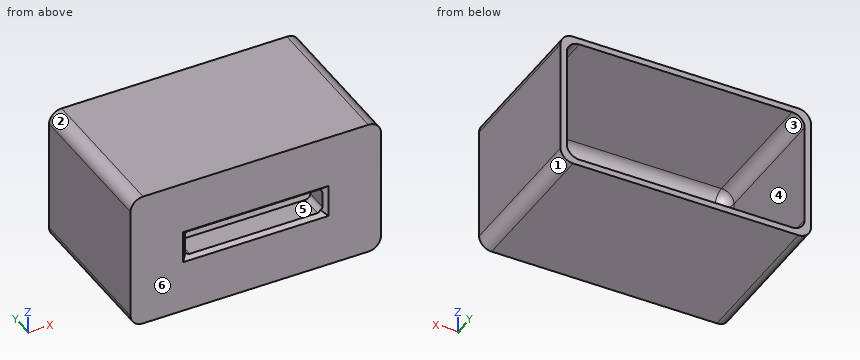
```python
from build123d import *

# Parameters (mm, degrees)
SKETCH1_W           = 200
SKETCH1_H           = 110
BOSS_EXTRUDE1_DEPTH = 6
SKETCH2_W           = 200
SKETCH2_H           = 110
SKETCH2_W_2         = 190
SKETCH2_H_2         = 100
BOSS_EXTRUDE2_DEPTH = 114
SKETCH3_W           = 110
SKETCH3_H           = 20
CUT_EXTRUDE1_DEPTH  = 256.139177705
SKETCH4_W           = 120
SKETCH4_H           = 30
SKETCH4_W_2         = 110
SKETCH4_H_2         = 20
BOSS_EXTRUDE3_DEPTH = 15
CHAMFER2_SIZE       = 3
FILLET1_R           = 10
FILLET2_R           = 4


with BuildPart() as part:
    # Sketch1 → Boss-Extrude1 (new body)
    with BuildSketch(Plane(origin=(0, 0, 0), x_dir=(1, 0, 0), z_dir=(0, 1, 0))):
        with Locations((100, 55)):
            Rectangle(SKETCH1_W, SKETCH1_H)
    extrude(amount=BOSS_EXTRUDE1_DEPTH)

    # Sketch2 → Boss-Extrude2 (add)
    with BuildSketch(Plane(origin=(0, 6, 0), x_dir=(1, 0, 0), z_dir=(0, 1, 0))):
        with Locations((100, 55)):
            Rectangle(SKETCH2_W, SKETCH2_H)
        with Locations((100, 55)):
            Rectangle(SKETCH2_W_2, SKETCH2_H_2, mode=Mode.SUBTRACT)
    extrude(amount=BOSS_EXTRUDE2_DEPTH)

    # Sketch3 → Cut-Extrude1 (cut, through all)
    with BuildSketch(Plane(origin=(0, 6, 0), x_dir=(1, 0, 0), z_dir=(0, 1, 0))):
        with Locations((100, 55)):
            Rectangle(SKETCH3_W, SKETCH3_H)
    extrude(amount=-CUT_EXTRUDE1_DEPTH, mode=Mode.SUBTRACT)

    # Sketch4 → Boss-Extrude3 (add)
    with BuildSketch(Plane(origin=(0, 6, 0), x_dir=(1, 0, 0), z_dir=(0, 1, 0))):
        with Locations((100, 55)):
            Rectangle(SKETCH4_W, SKETCH4_H)
        with Locations((100, 55)):
            Rectangle(SKETCH4_W_2, SKETCH4_H_2, mode=Mode.SUBTRACT)
    extrude(amount=BOSS_EXTRUDE3_DEPTH)

    # Chamfer2
    chamfer2_edges = [part.edges().sort_by_distance(p)[0] for p in [
        (45, 0, -55),
        (100, 0, -65),
        (155, 0, -55),
        (100, 0, -45),
    ]]
    chamfer(chamfer2_edges, length=CHAMFER2_SIZE)

    # Fillet1
    fillet1_edges = [part.edges().sort_by_distance(p)[0] for p in [
        (5, 6, -55),
        (100, 6, -5),
        (195, 6, -55),
        (100, 6, -105),
        (195, 63, -5),
        (195, 63, -105),
        (5, 63, -105),
        (5, 63, -5),
        (0, 60, -110),
        (200, 60, -110),
        (200, 60, 0),
        (0, 60, 0),
    ]]
    fillet(fillet1_edges, radius=FILLET1_R)

    # Fillet2
    fillet2_edges = [part.edges().sort_by_distance(p)[0] for p in [
        (100, 6, -70),
        (160, 13.5, -70),
        (40, 6, -55),
        (40, 13.5, -70),
        (100, 6, -40),
        (40, 13.5, -40),
        (160, 6, -55),
        (160, 13.5, -40),
        (155, 12, -45),
        (155, 12, -65),
        (45, 12, -65),
        (45, 12, -45),
    ]]
    fillet(fillet2_edges, radius=FILLET2_R)


solid = part.part
```
Part model, mm, in its own coordinate system. Face numbers are marked on the shaded views. A direction names the side the tool comes from. Coordinates: 2 decimals unless noted, no trailing zeros. Order: outer loops, then holes, each group sorted by start corner. A loop starts at its lowest first (then second) coordinate and runs counter-clockwise, first axis right, second up. Notation, with made-up numbers: (66.25, -21) -> (95.25, -21) arc R26 ccw to (95.25, 9) -> close; hole circle Ø9 at (11, 19). An arc over 180 degrees is marked (long way). Put each result on its own line as item: value. Start each with the question number.
(1) Probe line 1 along Z through (x, y) = (57, 15); line 2 along Z through (x, y) = (128, 88); line 3 along X through (y, z) = (59, -71.5). List the from-to ranges inside material, lowest first. Write a range as [from, to].
(2) Which spindle directions (+Z, -Z, +X, -X, +Y, -Y) get a long thin tool onto all of the face, cutting with end or side? Do the marked faces 4, 5 and 6. Say none if no direction does.
(3) Band-saw the part on B-B (y = 101). Give the cut face in (x, z).
(4) Mould opens along X. For the marked faces 1, 2 and 3 say: pulls with the +X half, pulls with the -X half, needs draft (parallel to the pull), parting line crosses it, or undercut.
(5) Band-saw the part on D-D (x = 173). Give the cut face in (y, z).
(6) Band-saw the part on A-A (x = 92.5). Give the cut face in (y, z), then the cut area to 3 significant figures.
(7) Band-saw the part on C-C (z = -86.5). Give the cut face in (x, y), then the cut area to 3 significant figures.
Determined:
1. line 1: z = [-110, -104.95], [-70, -65], [-45, -40], [-5.05, 0]
1. line 2: z = [-110, -105], [-5, 0]
1. line 3: x = [0, 5], [195, 200]
2. face 4: +Y
2. face 5: +Y, -Y
2. face 6: +Z, -Z, +X, -X, -Y
3. outline: (0, -100) arc R10 ccw to (10, -110) -> (190, -110) arc R10 ccw to (200, -100) -> (200, -10) arc R10 ccw to (190, 0) -> (10, 0) arc R10 ccw to (0, -10) -> close; hole (5, -95) arc R10 ccw to (15, -105) -> (185, -105) arc R10 ccw to (195, -95) -> (195, -15) arc R10 ccw to (185, -5) -> (15, -5) arc R10 ccw to (5, -15) -> close
4. face 1: pulls with the +X half
4. face 2: pulls with the -X half
4. face 3: undercut
5. outline: (0, -110) -> (120, -110) -> (120, -105) -> (16, -105) arc R10 cw to (6, -95) -> (6, -15) arc R10 cw to (16, -5) -> (120, -5) -> (120, 0) -> (0, 0) -> close
6. outline: (0, -110) -> (120, -110) -> (120, -105) -> (16, -105) arc R10 cw to (6, -95) -> (6, -74) arc R4 cw to (10, -70) -> (21, -70) -> (21, -65) -> (3, -65) -> (0, -68) -> close; (0, -42) -> (3, -45) -> (21, -45) -> (21, -40) -> (10, -40) arc R4 cw to (6, -36) -> (6, -15) arc R10 cw to (16, -5) -> (120, -5) -> (120, 0) -> (0, 0) -> close
6. area: 1,870 mm²
7. outline: (0, 0) -> (200, 0) -> (200, 120) -> (195, 120) -> (195, 16) arc R10 cw to (185, 6) -> (15, 6) arc R10 cw to (5, 16) -> (5, 120) -> (0, 120) -> close
7. area: 2,380 mm²
